Input: part model. Units: mm. Frame: model coordinates. Round coordinates to 2 decimals unless told otherwise and drop trailing zeros. Loops run counter-clockwise (first coordinate to the right, second up) from the corner with the lowest first, then second, coordinate; pieces in that order, holes last. Notation, with made-up numbers: (75.25, 33.5) -> (131.25, 33.5) arc R21 cw to (131.25, 47.5) -> close; hole circle Ø4 at (-18, 35). An arc over 180 degrees is marked (long way). Answer as a JSON object with one key per item and string values.
```python
from build123d import *

# Parameters (mm, degrees)
SKETCH1_W           = 50
SKETCH1_H           = 10
BOSS_EXTRUDE1_DEPTH = 154
SKETCH2_R           = 4
CUT_EXTRUDE1_DEPTH  = 157.336176236


with BuildPart() as part:
    # Sketch1 → Boss-Extrude1 (new, symmetric)
    with BuildSketch(Plane(origin=(0, 0, 0), x_dir=(1, 0, 0), z_dir=(0, 1, 0))):
        Rectangle(SKETCH1_W, SKETCH1_H)
    extrude(amount=BOSS_EXTRUDE1_DEPTH, both=True)

    # Sketch2 → Cut-Extrude1 (cut, through all)
    with BuildSketch(Plane(origin=(0, 0, -5), x_dir=(-1, 0, 0), z_dir=(0, 0, -1))):
        with Locations((0, -129)):
            Circle(SKETCH2_R)
        with Locations(Location((0, 129, 0), (0, 0, 180))):
            Circle(SKETCH2_R)
    extrude(amount=-CUT_EXTRUDE1_DEPTH, mode=Mode.SUBTRACT)


solid = part.part
```
1) Ray query, probe 1 along Y at (x, z) = (0, 0.5); probe 2 along X at (y, z) = (129, 2.25); probe 3 along X at (y, z) = (-131, -2). Return the intervals inside material, ascending.
Output:
{"probe 1": "y = -154 to -133, -125 to 125, 133 to 154", "probe 2": "x = -25 to -4, 4 to 25", "probe 3": "x = -25 to -3.46, 3.46 to 25"}
2) Section B-B, the plane x = 0. Output: boundary loops of the cut face in (y, z).
Output:
{"outline": "(-154, -5) -> (-133, -5) -> (-133, 5) -> (-154, 5) -> close; (-125, -5) -> (125, -5) -> (125, 5) -> (-125, 5) -> close; (133, -5) -> (154, -5) -> (154, 5) -> (133, 5) -> close"}
3) Section A-A, the plane y = -129. Output: boundary loops of the cut face in (x, z), plus the area to 3 significant figures.
Output:
{"outline": "(-25, -5) -> (-4, -5) -> (-4, 5) -> (-25, 5) -> close; (4, -5) -> (25, -5) -> (25, 5) -> (4, 5) -> close", "area": "420 mm^2"}
4) Draft query along X for faces 1 (the face through (-0.521, 125.034, -0.07)), 2 (the face through (25, 2, 0)), 3 (the face through (0, 2, -5)). Return one class per face: +X half, -X half, draft (parallel to the pull), parting line (faces both ways), or undercut.
Output:
{"face 1": "undercut", "face 2": "+X half", "face 3": "draft"}
5) Contact query for a flat-ended pin moving along its axis: P1, Ø5, axis at x = 0, y = -129, coming from the -Z side. Output: stop coordinate, or through.
Output:
{"P1": "passes through"}
